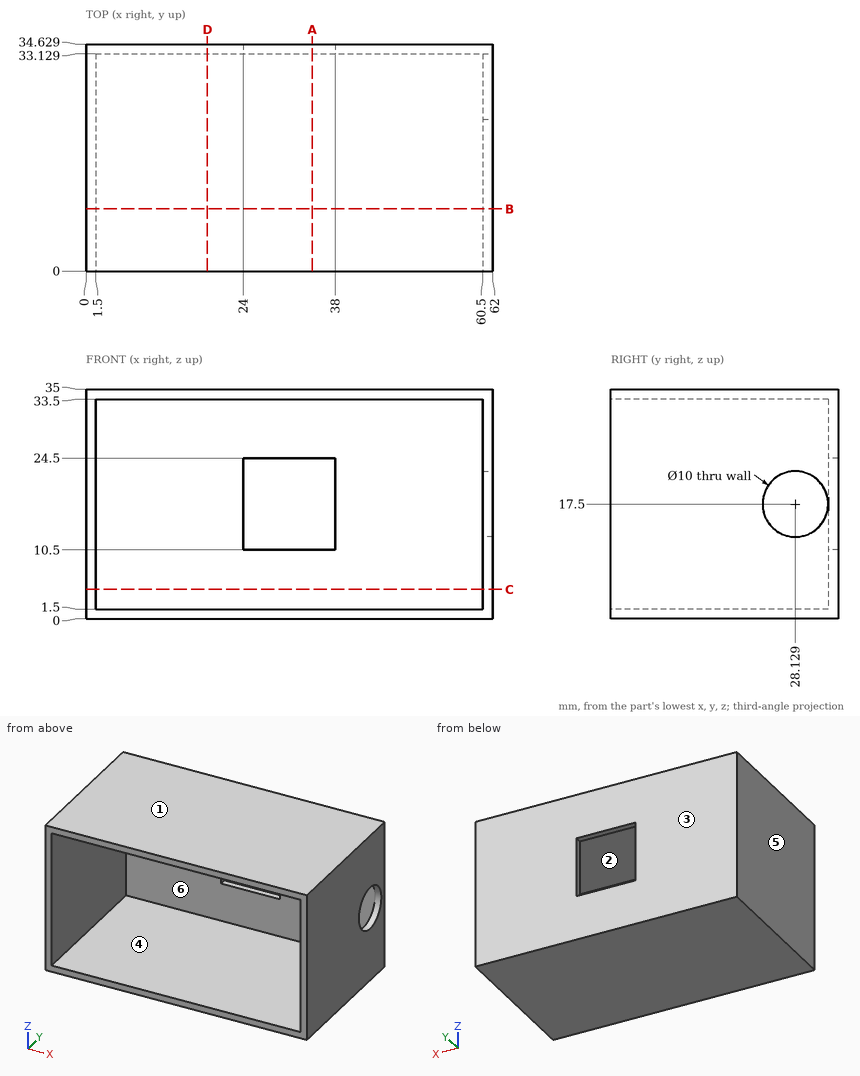
Drawing for the job (mm, zero at the part's lowest x, y, z). A direction names the side the tool comes from. Give positions to 0.01 mm unless a question says otherwise; leave off trailing zeros. Loops run counter-clockwise (first coordinate to the right, second up) from the corner with the lowest first, then second, coordinate; pieces in that order, holes last.
(1) Band-saw the part on B-B (y = 9.5). Write the cut outline in (x, z), and give its area (3 significant figures).
Return value:
outline: (0, 0) - (62, 0) - (62, 35) - (0, 35) - close; hole (1.5, 1.5) - (60.5, 1.5) - (60.5, 33.5) - (1.5, 33.5) - close
area: 282 mm2
(2) Band-saw the part on A-A (x = 34.5). Write the cut outline in (y, z).
Return value:
outline: (0, 0) - (34.63, 0) - (34.63, 10.5) - (33.13, 10.5) - (33.13, 1.5) - (0, 1.5) - close; (0, 33.5) - (33.13, 33.5) - (33.13, 24.5) - (34.63, 24.5) - (34.63, 35) - (0, 35) - close
(3) Drill centre lines: line 1 along Z through (x, y) = (19.5, 31.5); line 2 along X through (y, z) = (18.5, 8.5); line 3 along Y through (x, z) = (61.45, 17.5). Where is each one in solid material? Low to high.
Return value:
line 1: z = 0 to 1.5, 33.5 to 35
line 2: x = 0 to 1.5, 60.5 to 62
line 3: y = 0 to 23.13, 33.13 to 34.63
(4) Band-saw the part on D-D (x = 18.5). Write the cut outline in (y, z).
Return value:
outline: (0, 0) - (34.63, 0) - (34.63, 35) - (0, 35) - (0, 33.5) - (33.13, 33.5) - (33.13, 1.5) - (0, 1.5) - close
(5) 3-axis set-ups, long thin cutter, end or side, ignore diameter. For the marked faces 1 and 2: which of +Z, -Z, +X, -X, +Y, -Y reach the whole face in a straight line?
Return value:
face 1: +Z, +X, -X, +Y, -Y
face 2: -Y
(6) Pull direction X, two halves, no side cores. Call the marked faces 3, 4, 5 and 6: pulls with the +X half, pulls with the -X half, needs draft (parallel to the pull), parting line crosses it, or undercut.
Return value:
face 3: needs draft
face 4: undercut
face 5: pulls with the -X half
face 6: undercut
(7) Band-saw the part on C-C (z = 4.5). Write the cut outline in (x, y).
Return value:
outline: (0, 0) - (1.5, 0) - (1.5, 33.13) - (60.5, 33.13) - (60.5, 0) - (62, 0) - (62, 34.63) - (0, 34.63) - close
(8) Pin check, flat tips, straight feed: pin 1 (12 mm diameter, centred on x = 49, z = 23, fed in from -Y); pin 2 (6 mm diameter, centred on y = 28.13, z = 17.5, fed in from +X). Stop position of each tip, or through.
Return value:
pin 1: stops at y = 33.13
pin 2: stops at x = 1.5
